from build123d import *

# Parameters (mm, degrees)
BOX_W          = 20
BOX_H          = 30
BOX_DEPTH      = 40
FILLET_R       = 5
CYLINDER_R     = 6.4
CYLINDER_DEPTH = 40
BOX001_W       = 40
BOX001_H       = 40
BOX001_DEPTH   = 40
FILLET001_R    = 4


with BuildPart() as obj1:
    # Box → Box (new body)
    with BuildSketch(Plane(origin=(18.5, -15, 0), x_dir=(1, 0, 0), z_dir=(0, 0, 1))):
        with Locations((10, 15)):
            Rectangle(BOX_W, BOX_H)
    extrude(amount=BOX_DEPTH)

    # Fillet
    fillet_edges = [obj1.edges().sort_by_distance(p)[0] for p in [
        (18.5, -15, 20),
        (18.5, 15, 20),
    ]]
    fillet(fillet_edges, radius=FILLET_R)


with BuildPart() as cylinder:
    # Cylinder → Cylinder (new body)
    with BuildSketch(Plane.XY):
        Circle(CYLINDER_R)
    extrude(amount=CYLINDER_DEPTH)


with BuildPart() as fusion001:
    # Box001 → Box001 (new body)
    with BuildSketch(Plane(origin=(-20, -20, 20), x_dir=(1, 0, 0), z_dir=(0, 0, 1))):
        with Locations((20, 20)):
            Rectangle(BOX001_W, BOX001_H)
    extrude(amount=BOX001_DEPTH)

    # Fusion: union Cylinder
    add(cylinder.part)

    # Fusion001: union obj1
    add(obj1.part)


with BuildPart() as fillet001:
    # Cone → Cone (revolve)
    with BuildSketch(Plane.XZ):
        Polygon((0, 0), (30, 0), (1, 40), (0, 40), align=None)
    revolve(axis=Axis((0, 0, 0), (0, 0, 1)))

    # Cut: cut Fusion001
    add(fusion001.part, mode=Mode.SUBTRACT)

    # Fillet001
    fillet001_edges = [fillet001.edges().sort_by_distance(p)[0] for p in [
        (18.5, -5.247536, 14.855397),
        (20.110238, -13.675529, 7.835067),
        (20.110238, 13.675529, 7.835067),
        (18.5, 5.247536, 14.855397),
    ]]
    fillet(fillet001_edges, radius=FILLET001_R)


solid = fillet001.part
Work out the finished part from the listing and answer in its coordinate system (mm). A direction names the side the tool comes from. Coordinates: 2 decimals unless noted, no trailing zeros. Write each loop counter-clockwise with the first axis right and the second up, starting at its lowest first coordinate (ties: lowest second). Pieces come first, ordered by that corner, then holes. Notation, with made-up numbers: M 87.5,30.25 L 135.5,30.25 A25 cw 135.5,52.25 Z; hole C -5,25 d9. An arc over 180 degrees is marked long. Use one line per item in the form item = value. Start each with the question number.
1. A tool of negligible diameter and unlimited length cuts with its end or side. For faces 4 (the face through (18.824, 11.77, 4.077)), 5 (the face through (7, 0, 20)), from which of +Z, -Z, +X, -X, +Y, -Y can it reach the whole face along a straight path? Write none if from no direction.
2. The part is cut by section A-A (x = 0). Give the vertices of the cut face in (y, z), plus the area to 3 significant figures.
3. The mould has two halves that part along X. Classify faces 1 (the face through (-5.08, -3.89, 9.86)), 2 (the face through (-9, 0, 0)), 3 (the face through (-16.19, 0.71, 19.03)): released by +X, released by -X, zero draft, split by the parting line, or undercut.
4. Straight lines are drawn through the part: probe 1 along X at (y, z) = (5, 8.5) (3 decimals); probe 2 along Y at (x, z) = (2.5, 10.75); probe 3 along X at (y, z) = (3.5, 19.25). For each, find the intervals that lie inside material, in ascending order. Write a range as from..to.
5. Each of these flat-tipped pins is pushed along its axis until it touches: P1, Ø1, axis at y = -5, z = 3, coming from the -X side; P2, Ø1, axis at x = -19, z = 12, coming from the -Y side; P3, Ø10, axis at x = -19, z = 10, coming from the +Y side; P4, Ø12, axis at x = -1, y = 8.5, coming from the -Z side. Where does it stop, or does it pass through?
Evaluation:
q1.face_4 = +Z, -Z, +X
q1.face_5 = +Z, +X, -X, +Y, -Y
q2.outline = M -30,0 L -6.4,0 L -6.4,20 L -15.5,20 Z; M 6.4,0 L 30,0 L 15.5,20 L 6.4,20 Z
q2.area = 654 mm^2
q3.face_1 = undercut
q3.face_2 = zero draft
q3.face_3 = split by the parting line
q4.probe_1 = -23.307..-3.995, 3.995..18.5
q4.probe_2 = -22.07..-5.89, 5.89..22.07
q4.probe_3 = -15.66..-5.36, 5.36..15.66
q5.P1 = -27.75
q5.P2 = -10.82
q5.P3 = 20.06
q5.P4 = 0
